Here's how the part is built. I have some questions about the finished solid (model axes, mm). A direction names the side the tool comes from. Round coordinates to 2 decimals unless told otherwise and drop trailing zeros. Loops run counter-clockwise (first coordinate to the right, second up) from the corner with the lowest first, then second, coordinate; pieces in that order, holes last. Notation, with made-up numbers: M -28,88.5 L 11,88.5 A17 cw 11,95.5 Z; hole C 6,-35 d7. An arc over 180 degrees is marked long. Write each question's results on one line, items separated by ' | '. Start each with the question number.
```python
from build123d import *

# Parameters (mm, degrees)
SKETCH_1_W                    = 180
SKETCH_1_H                    = 180
EXTRUDE_1_DEPTH               = 15
HOLE_WIZARD_4_8_1_D           = 6.5
HOLE_WIZARD_4_8_1_CBORE_D     = 11
HOLE_WIZARD_4_8_1_CBORE_DEPTH = 6.5
HOLE_WIZARD_6_0_6_1_D         = 6
HOLE_WIZARD_4_8_2_D           = 9
HOLE_WIZARD_4_8_2_CBORE_D     = 15
HOLE_WIZARD_4_8_2_CBORE_DEPTH = 9


with BuildPart() as part:
    # 草图1 → 凸台-拉伸1 (new body)
    with BuildSketch(Plane.XY):
        Rectangle(SKETCH_1_W, SKETCH_1_H)
    extrude(amount=EXTRUDE_1_DEPTH)

    # 打孔尺寸根据内六角花形圆柱头螺钉-4.8级的类型1 (through all)
    with Locations(Plane(origin=(-61, 61, 15), x_dir=(1, 0, 0), z_dir=(0, 0, 1))):
        with Locations((0, 0), (96, 0), (26, 0), (0, -122), (26, -122), (96, -122), (122, -122), (122, 0)):
            CounterBoreHole(HOLE_WIZARD_4_8_1_D / 2, HOLE_WIZARD_4_8_1_CBORE_D / 2, HOLE_WIZARD_4_8_1_CBORE_DEPTH)

    # Ø6.0 (6) 直径孔1 (through all)
    with Locations(Plane(origin=(0, 61, 15), x_dir=(1, 0, 0), z_dir=(0, 0, 1))):
        with Locations((0, 0), (0, -122)):
            Hole(HOLE_WIZARD_6_0_6_1_D / 2)

    # 打孔尺寸根据内六角花形圆柱头螺钉-4.8级的类型2 (through all)
    with Locations(Plane(origin=(60, 75, 0), x_dir=(-1, 0, 0), z_dir=(0, 0, -1))):
        with Locations((0, 0), (60, 0), (120, 0), (120, -150), (60, -150), (0, -150)):
            CounterBoreHole(HOLE_WIZARD_4_8_2_D / 2, HOLE_WIZARD_4_8_2_CBORE_D / 2, HOLE_WIZARD_4_8_2_CBORE_DEPTH)


solid = part.part
```
1. I want a section at C-C on x = 0. List the corners of the cut face in (y, z) for me.
2. I need wall thicknesses on line 1 along Y through (x, z) = (0, 11.35); line 2 along Y through (x, z) = (35.5, 12.75); line 3 along Y through (x, z) = (-56, 1.5). Which ranges of each line are inside material? Lowest first, please.
3. Which directions (+Z, -Z, +X, -X, +Y, -Y) give clear straight access to the entire face, cutting with the end or side of a thin tool? Please do faces 4 (the face through (-65.05, -57.28, 11.8)), 5 (the face through (-3.461, -81.654, 4.437)), 6 (the face through (-0.59, -70.54, 12.04)).
4. For pin 1 (5.5 mm diameter, centred on x = 58.5, y = 61.5, fed in from +Z), with a flat end and sliding along its axis, tell me the tip position at first contact or that it passes through.
5. If we mould it in two halves opening along X, with no side actions, what happens to faces 1 (the face through (-1, -90, 7)), 2 (the face through (-90, -1, 7)), 3 (the face through (63.395, 63.197, 4.19))? For each: released by +X, released by -X, zero draft, split by the parting line, or undercut.
6. I want a section at B-B on z = 3.75. Count the separate pieces of the cut face and the enclosed holes in it, plus the area to 3 significant figures.
7. I want a section at A-A on y = 75. List the corners of the cut face in (x, z) for me.
Outcome:
1) outline: M -90,0 L -82.5,0 L -82.5,9 L -79.5,9 L -79.5,15 L -90,15 Z; M -70.5,9 L -67.5,9 L -67.5,0 L -64,0 L -64,15 L -70.5,15 Z; M -58,0 L 58,0 L 58,15 L -58,15 Z; M 64,0 L 67.5,0 L 67.5,9 L 70.5,9 L 70.5,15 L 64,15 Z; M 79.5,9 L 82.5,9 L 82.5,0 L 90,0 L 90,15 L 79.5,15 Z
2) line 1: -90 to -79.5, -70.5 to -64, -58 to 58, 64 to 70.5, 79.5 to 90 | line 2: -90 to -66.48, -55.52 to 55.52, 66.48 to 90 | line 3: -90 to -81.34, -68.66 to 68.66, 81.34 to 90
3) face 4: +Z | face 5: -Z | face 6: +Z, -Z
4) pin 1: z = 8.5
5) face 1: zero draft | face 2: released by -X | face 3: undercut
6) separate pieces: 1 | enclosed holes: 16 | area: 31,000 mm2
7) outline: M -90,0 L -67.5,0 L -67.5,9 L -64.5,9 L -64.5,15 L -90,15 Z; M -55.5,9 L -52.5,9 L -52.5,0 L -7.5,0 L -7.5,9 L -4.5,9 L -4.5,15 L -55.5,15 Z; M 4.5,9 L 7.5,9 L 7.5,0 L 52.5,0 L 52.5,9 L 55.5,9 L 55.5,15 L 4.5,15 Z; M 64.5,9 L 67.5,9 L 67.5,0 L 90,0 L 90,15 L 64.5,15 Z
